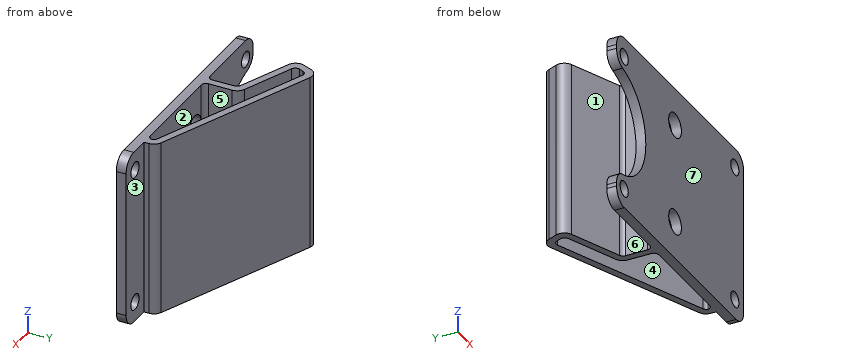
from build123d import *

# Parameters (mm, degrees)
F1_DEPTH     = 36
F2_T         = -1.5
F3_R         = 1.6
F4_DEPTH     = 1.5
F5_R         = 1.6
F6_DEPTH     = 5
F7_DEPTH     = 0.5
F8_DEPTH     = 0.5
F9_R         = 3
F10_T1_DEPTH = 36
F11_R        = 2
F5_R_2       = 2.5
F12_DEPTH    = 5


# Not quite as in the source:
# - a fillet or chamfer that OpenCascade refuses, or shapes differently, is made with other operations: its cross-section is extruded or revolved along the edge and cut away or added


with BuildPart() as f1:
    # F0 (on Top) → F1 (new body)
    with BuildSketch(Plane.XY):
        Polygon((-12, 0), (20, 0), (20, 1.5), (13, 1.5), (13, 4.3777777778), (-22.720401141, 19.0628315802), (-25, 13.5178613825), (-12, 8.1734169381), (-12, 1.5), (-30, 1.5), (-30, 0), align=None)
    extrude(amount=F1_DEPTH)

    # F2: a shell. OpenCascade refuses it in one call, so the cavity is built on its own and cut out:
    # the body offset inwards by the wall thickness, plus a prism from it out through each open face.
    f2_core = offset(f1.part, amount=F2_T, kind=Kind.INTERSECTION, mode=Mode.PRIVATE)
    f2_exits = [f2_core.faces().sort_by_distance(p)[0] for p in [
        (-5.203768, 6.959906, 34.5),
        (-5.203768, 6.959906, 1.5),
    ]]
    add(f2_core, mode=Mode.SUBTRACT)
    extrude(f2_exits, amount=-F2_T, mode=Mode.SUBTRACT)

    # F3 (on face) → F4 (cut)
    with BuildSketch(Plane(origin=(0, 1.5, 0), x_dir=(-1, 0, 0), z_dir=(0, 1, 0))):
        with Locations((-16.5, 32)):
            Circle(F3_R)
        with Locations((-16.5, 4)):
            Circle(F3_R)
    extrude(amount=-F4_DEPTH, mode=Mode.SUBTRACT)

    # F5 (on face) → F6 (cut)
    with BuildSketch(Plane.XZ):
        with Locations((-27, 32)):
            Circle(F5_R)
        with BuildLine():
            Line((-30, 29.5), (-30, 6.5))
            ThreePointArc((-30, 6.5), (-18.5, 18), (-30, 29.5))
        make_face()
        with Locations((-27, 4)):
            Circle(F5_R)
    extrude(amount=-F6_DEPTH, mode=Mode.SUBTRACT)

    # F7 (add): faces of the model
    f7_faces = [f1.faces().sort_by_distance(p)[0] for p in [
        (16.5, 1.5, 18),
        (-21, 1.5, 0.4024922359),
    ]]
    extrude(f7_faces, amount=F7_DEPTH)

    # F8 (add): a face of the model
    f8_faces = [f1.faces().sort_by_distance(p)[0] for p in [
        (0.5, 1.5, 18),
    ]]
    extrude(f8_faces, amount=F8_DEPTH)

    # F9
    f9_edges = [f1.edges().sort_by_distance(p)[0] for p in [
        (20, 1, 36),
        (20, 1, 0),
        (-30, 1, 0),
        (-30, 1, 36),
        (-30, 1, 6.5),
        (-30, 1, 29.5),
    ]]
    fillet(f9_edges, radius=F9_R)

    # F10: fillet of radius 1 on 8 edges, made by hand

    # F10_s2 → F10_t1 (join)
    with BuildSketch(Plane.XY):
        with BuildLine():
            ThreePointArc((-10.5, 3), (-10.2071067812, 2.2928932188), (-9.5, 2))
            Line((-9.5, 2), (-10.5, 2))
            Line((-10.5, 2), (-10.5, 3))
        make_face()
        with BuildLine():
            ThreePointArc((-22.1174237286, 13.954615363), (-22.6600526413, 14.4943748472), (-22.6620816337, 15.2597390224))
            Line((-22.6620816337, 15.2597390224), (-23.0423145109, 14.3348482402))
            Line((-23.0423145109, 14.3348482402), (-22.1174237286, 13.954615363))
        make_face()
        with BuildLine():
            ThreePointArc((-22.2836471604, 16.1802553088), (-21.7438876763, 16.7228842215), (-20.978523501, 16.7249132139))
            Line((-20.978523501, 16.7249132139), (-21.9034142833, 17.105146091))
            Line((-21.9034142833, 17.105146091), (-22.2836471604, 16.1802553088))
        make_face()
        with BuildLine():
            ThreePointArc((10.8802328772, 3.6274244806), (11.3307324711, 3.2592055599), (11.5, 2.7025336984))
            Line((11.5, 2.7025336984), (11.5, 3.3726313301))
            Line((11.5, 3.3726313301), (10.8802328772, 3.6274244806))
        make_face()
        with BuildLine():
            ThreePointArc((-13, 2), (-12.2928932188, 2.2928932188), (-12, 3))
            Line((-12, 3), (-12, 2))
            Line((-12, 2), (-13, 2))
        make_face()
        with BuildLine():
            ThreePointArc((-12, 7.5033193063), (-12.1692675289, 8.0599911678), (-12.6197671228, 8.4282100886))
            Line((-12.6197671228, 8.4282100886), (-12, 8.1734169381))
            Line((-12, 8.1734169381), (-12, 7.5033193063))
        make_face()
        with BuildLine():
            ThreePointArc((11.5, 3), (11.2071067812, 2.2928932188), (10.5, 2))
            Line((10.5, 2), (11.5, 2))
            Line((11.5, 2), (11.5, 3))
        make_face()
    extrude(amount=F10_T1_DEPTH)

    # F11
    f11_edges = [f1.edges().sort_by_distance(p)[0] for p in [
        (-25, 13.517861, 18),
        (-22.720401, 19.062832, 18),
        (13, 4.377778, 18),
        (-10.5, 9.178563, 18),
    ]]
    fillet(f11_edges, radius=F11_R)

    # F5 (on face) → F12 (cut)
    with BuildSketch(Plane.XZ):
        with Locations((-7, 28.25)):
            Circle(F5_R_2)
        with Locations((-7, 7.75)):
            Circle(F5_R_2)
    extrude(amount=-F12_DEPTH, mode=Mode.SUBTRACT)


solid = f1.part
Design review of the part built by this model. Coordinates are the model's own, in mm. Face numbers are marked on the shaded views. A direction names the side the tool comes from. Round coordinates to 2 decimals unless told otherwise and drop trailing zeros. Write each loop counter-clockwise with the first axis right and the second up, starting at its lowest first coordinate (ties: lowest second). Pieces come first, ordered by that corner, then holes. Notation, with made-up numbers: (-30.75, -24.75) -> (3.25, -24.75) arc R19 cw to (3.25, 1.25) -> close; hole circle Ø9 at (55, 78). An arc over 180 degrees is marked (long way). One line per item, written item: value. Start each with the question number.
Q1. Add section A-A (x = -7). Give the boundary of the cut face in (y, z).
Q2. Add section C-C (z = 19.5). Give the boundary of the cut face in (x, y).
Q3. Add section D-D (x = 2). Give the boundary of the cut face in (y, z).
Q4. To check wall thickness, follow probe 1 along Z at (x, y) = (16.5, 1.15); probe 2 along Z at (x, y) = (-7, 1.1); probe 3 along Z at (x, y) = (-27, 1.1). State the ranges of each line that lie inside material, in increasing order.
Q5. Insertion check: P1, Ø1.5, axis at x = -18.5, z = 26.5, coming from the +Y side; P2, Ø8, axis at x = 11, z = 5.5, coming from the +Y side; P3, Ø4, axis at y = 15.5, z = 21.5, coming from the -X side. Each pin has a flat end and moves straight along its axis. Give the tip position at first contact, or say it passes through.
Q6. Add section B-B (y = 11.5). Give the boundary of the cut face in (x, z).
Q7. The part is to be moulded in two halves that separate along X. For the marked faces 4, 5, 6 and 7, say which applies: pulls with the +X half, pulls with the -X half, needs draft (parallel to the pull), parting line crosses it, or undercut.
Q8. Tool access review of the marked faces 1, 2 and 3: name each direction out of +Z, -Z, +X, -X, +Y, -Y from which nothing blocks a thin tool from reaching the whole face with its end or side.
Response:
1. outline: (0, 0) -> (2, 0) -> (2, 5.25) -> (0, 5.25) -> close; (0, 10.25) -> (2, 10.25) -> (2, 25.75) -> (0, 25.75) -> close; (0, 30.75) -> (2, 30.75) -> (2, 36) -> (0, 36) -> close; (10.98, 0) -> (12.6, 0) -> (12.6, 36) -> (10.98, 36) -> close
2. outline: (-24.24, 15.37) arc R2 ccw to (-23.15, 12.76) -> (-12.62, 8.43) arc R1 cw to (-12, 7.5) -> (-12, 3) arc R1 cw to (-13, 2) -> (-18.6, 2) -> (-18.6, 0) -> (20, 0) -> (20, 2) -> (13, 2) -> (13, 3.04) arc R2 ccw to (11.76, 4.89) -> (-20.87, 18.3) arc R2 ccw to (-23.48, 17.21) -> close; hole (-22.66, 15.26) arc R1 ccw to (-22.12, 13.95) -> (-11.74, 9.69) arc R2 cw to (-10.5, 7.84) -> (-10.5, 3) arc R1 ccw to (-9.5, 2) -> (10.5, 2) arc R1 ccw to (11.49, 2.85) arc R1 ccw to (10.88, 3.63) -> (-20.98, 16.72) arc R1 ccw to (-22.28, 16.18) -> close
3. outline: (0, 0) -> (2, 0) -> (2, 36) -> (0, 36) -> close; (7.28, 0) -> (8.9, 0) -> (8.9, 36) -> (7.28, 36) -> close
4. probe 1: z = 0 to 2.4, 5.6 to 30.4, 33.6 to 36
4. probe 2: z = 0 to 5.25, 10.25 to 25.75, 30.75 to 36
4. probe 3: z = 0 to 2.4, 5.6 to 6.9, 29.1 to 30.4, 33.6 to 36
5. P1: stops at y = 17.64
5. P2: stops at y = 6.84
5. P3: stops at x = -24.39
6. outline: (-20.09, 0) -> (-16.15, 0) -> (-16.15, 36) -> (-20.09, 36) -> close; (-8.27, 0) -> (-4.32, 0) -> (-4.32, 36) -> (-8.27, 36) -> close
7. face 4: undercut
7. face 5: undercut
7. face 6: pulls with the -X half
7. face 7: needs draft
8. face 1: +Z, -Z, -X
8. face 2: +Z, -Z
8. face 3: +Z, -Z, +X, +Y
